The listing builds one solid part. Answer for the finished solid, in the listing's coordinates (mm). Round coordinates to 2 decimals unless told otherwise and drop trailing zeros. Write each loop counter-clockwise with the first axis right and the second up, starting at its lowest first coordinate (ties: lowest second). Pieces come first, ordered by that corner, then holes. Notation, with made-up numbers: (-18.75, -26.5) - (17.25, -26.5) arc R25 cw to (17.25, 3.5) - close; hole circle Ø9 at (74, 27.25). An arc over 180 degrees is marked (long way). Return JSON: item names as keys, results as strings. Group by question number.
(1) Each of these flat-tipped pins is pushed along its axis until it touches: pin 1 (16 mm diameter, centred on y = -128.6, z = 21.69, fed in from +X); pin 2 (6 mm diameter, centred on x = 12.7, y = -742.73, fed in from +Z); pin 3 (8 mm diameter, centred on y = -1296.87, z = 21.69, fed in from +X). Where does it stop, or does it pass through?
(2) Section A-A, the plane y = -855.5 is taken. Write down the section's boundary in (x, z).
(3) Find the intervals of material crossed by line 1 along X through (y, z) = (-107, -19.5); line 2 along Z through (x, y) = (8, -306); line 3 along X through (y, z) = (-1320.5, -32), in increasing order. Write a range as [from, to].
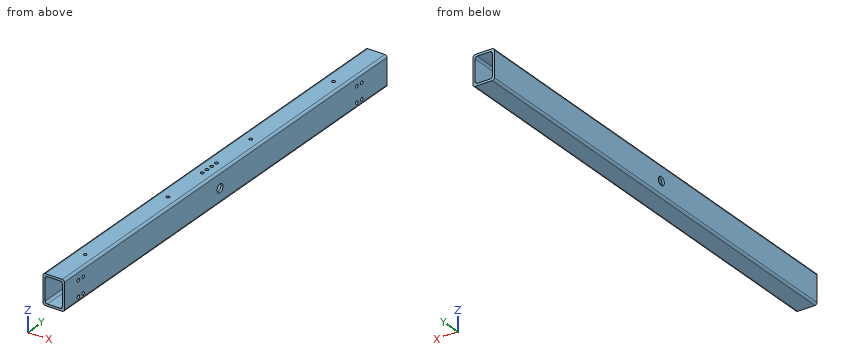
```python
from build123d import *

# Parameters (mm, degrees)
F1_DEPTH = 1377.117
F2_R     = 5
F3_DEPTH = 25
F4_R     = 5
F5_DEPTH = 25
F6_R     = 12.5
F7_DEPTH = 63.501


with BuildPart() as f1:
    # F0 (on Front) → F1 (new body)
    with BuildSketch(Plane.XZ):
        with BuildLine():
            Line((38.100001, 49.391132), (-12.699999, 49.391132))
            ThreePointArc((-12.699999, 49.391132), (-17.190127, 47.53126), (-19.049999, 43.041132))
            Line((-19.049999, 43.041132), (-19.049999, -33.158868))
            ThreePointArc((-19.049999, -33.158868), (-17.190127, -37.648996), (-12.699999, -39.508868))
            Line((-12.699999, -39.508868), (38.100001, -39.508868))
            ThreePointArc((38.100001, -39.508868), (42.590129, -37.648996), (44.450001, -33.158868))
            Line((44.450001, -33.158868), (44.450001, 43.041132))
            ThreePointArc((44.450001, 43.041132), (42.590129, 47.53126), (38.100001, 49.391132))
        make_face()
        with BuildLine():
            ThreePointArc((-12.699999, 36.691132), (-10.840127, 41.18126), (-6.349999, 43.041132))
            Line((-6.349999, 43.041132), (31.750001, 43.041132))
            ThreePointArc((31.750001, 43.041132), (36.240129, 41.18126), (38.100001, 36.691132))
            Line((38.100001, 36.691132), (38.100001, -26.808868))
            ThreePointArc((38.100001, -26.808868), (36.240129, -31.298996), (31.750001, -33.158868))
            Line((31.750001, -33.158868), (-6.349999, -33.158868))
            ThreePointArc((-6.349999, -33.158868), (-10.840127, -31.298996), (-12.699999, -26.808868))
            Line((-12.699999, -26.808868), (-12.699999, 36.691132))
        make_face(mode=Mode.SUBTRACT)
    extrude(amount=F1_DEPTH)

    # F2 (on face) → F3 (cut)
    with BuildSketch(Plane.YZ.offset(44.450001)):
        with Locations((-1317.667, 21.691132)):
            Circle(F2_R)
        with Locations((-1317.667, -24.508868)):
            Circle(F2_R)
        with Locations((-1296.867, 21.691132)):
            Circle(F2_R)
        with Locations((-1296.867, -24.508868)):
            Circle(F2_R)
        with Locations((-128.6, 21.691132)):
            Circle(F2_R)
        with Locations((-128.6, -24.508868)):
            Circle(F2_R)
        with Locations((-107.8, 21.691132)):
            Circle(F2_R)
        with Locations((-107.8, -24.508868)):
            Circle(F2_R)
    extrude(amount=-F3_DEPTH, mode=Mode.SUBTRACT)

    # F4 (on face) → F5 (cut)
    with BuildSketch(Plane.XY.offset(49.391132)):
        with Locations((12.700001, -1242.477)):
            Circle(F4_R)
        with Locations((12.700001, -889.32)):
            Circle(F4_R)
        with Locations((12.700001, -536.147)):
            Circle(F4_R)
        with Locations((12.700001, -182.975)):
            Circle(F4_R)
        with Locations((12.700001, -742.7265)):
            Circle(F4_R)
        with Locations((12.700001, -722.7265)):
            Circle(F4_R)
        with Locations((12.700001, -702.7265)):
            Circle(F4_R)
        with Locations((12.700001, -682.7265)):
            Circle(F4_R)
    extrude(amount=-F5_DEPTH, mode=Mode.SUBTRACT)

    # F6 (on face) → F7 (cut, through all)
    with BuildSketch(Plane(origin=(-19.049999, 0, 0), x_dir=(0, -1, 0), z_dir=(-1, 0, 0))):
        with Locations((712.726, 2.691132)):
            Circle(F6_R)
    extrude(amount=-F7_DEPTH, mode=Mode.SUBTRACT)


solid = f1.part
```
Working result:
{
 "1": {"pin 1": "stops at x = 44.45", "pin 2": "stops at z = -33.16", "pin 3": "stops at x = -12.7"},
 "2": {"outline": "(-19.05, -33.16) arc R6.35 ccw to (-12.7, -39.51) - (38.1, -39.51) arc R6.35 ccw to (44.45, -33.16) - (44.45, 43.04) arc R6.35 ccw to (38.1, 49.39) - (-12.7, 49.39) arc R6.35 ccw to (-19.05, 43.04) - close; hole (-12.7, -26.81) arc R6.35 ccw to (-6.35, -33.16) - (31.75, -33.16) arc R6.35 ccw to (38.1, -26.81) - (38.1, 36.69) arc R6.35 ccw to (31.75, 43.04) - (-6.35, 43.04) arc R6.35 ccw to (-12.7, 36.69) - close"},
 "3": {"line 1": "x = [-19.05, -12.7], [38.1, 44.45]", "line 2": "z = [-39.51, -33.16], [43.04, 49.39]", "line 3": "x = [-19.05, -10.01], [35.41, 44.45]"}
}
